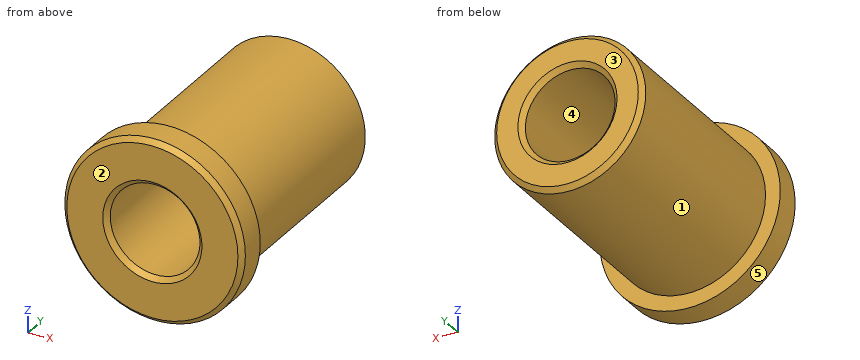
from build123d import *

# Parameters (mm, degrees)
CHAMFER1_SIZE = 0.25


with BuildPart() as part:
    # Sketch1 → Revolve1 (revolve)
    with BuildSketch(Plane.XY):
        Polygon((-2.375, 0), (-2.375, 12.7125), (-4, 12.7125), (-4, 1.6), (-4.78, 1.6), (-4.78, 0), align=None)
    revolve(axis=Axis((0, 0, 0), (0, 1, 0)))

    # Chamfer1
    chamfer1_edges = [part.edges().sort_by_distance(p)[0] for p in [
        (4.78, 0, 0),
        (4, 12.7125, 0),
        (2.375, 12.7125, 0),
        (2.375, 0, 0),
    ]]
    chamfer(chamfer1_edges, length=CHAMFER1_SIZE)


solid = part.part
Source: CAD feature listing. Evaluate the final solid. Frame: model axes, mm. Face numbers are marked on the shaded views. A direction names the side the tool comes from. Round coordinates to 2 decimals unless told otherwise and drop trailing zeros. Write each loop counter-clockwise with the first axis right and the second up, starting at its lowest first coordinate (ties: lowest second). Pieces come first, ordered by that corner, then holes. Notation, with made-up numbers: M 68,43.5 L 111,43.5 A16 ccw 111,73.5 Z; hole C -37,65 d11. An arc over 180 degrees is marked long. One line per item, written item: value. Start each with the question number.
Item 1: Pin query (flat end, axial travel): pin 1 (1 mm diameter, centred on x = -3, y = 7.5, fed in from +Z). Return the tip coordinate at first contact, or that it passes through.
Item 2: Ray query, L1, parallel to Z at x = 0, y = 8.25 (3 decimals); L2, parallel to Z at x = -1.5, y = 10.5. Return the intervals inside material, ascending. Write a range as from..to.
Item 3: Section query C-C (y = 11). Return the cut outline in (x, z) (3 decimals).
Item 4: Set-up query: the marked faces 1 and 2. Return all of +Z, -Z, +X, -X, +Y, -Y with unobstructed straight access to the full face (end or side cutting, diameter ignored); none if empty.
Item 5: Mould query, pull axis Z, two halves, no side actions, for the marked faces 3, 4 and 5. Classes: pulls with the +Z half, pulls with the -Z half, needs draft (parallel to the pull), parting line crosses it, or undercut.
Result set:
1. pin 1: stops at z = 3.12
2. L1: z = -4..-2.375, 2.375..4
2. L2: z = -3.71..-1.84, 1.84..3.71
3. outline: C 0,0 d8; hole C 0,0 d4.75
4. face 1: +Y
4. face 2: +Z, -Z, +X, -X, -Y
5. face 3: needs draft
5. face 4: undercut
5. face 5: parting line crosses it
